Print and shaded views of the part. All mm, measured from the part's lowest x, y and z. Round coordinates to 2 decimals unless told otherwise and drop trailing zeros. Loops run counter-clockwise (first coordinate to the right, second up) from the corner with the lowest first, then second, coordinate; pieces in that order, holes last. Notation, with made-up numbers: (46.5, 58) - (66.5, 58) arc R27 ccw to (66.5, 92) - close; hole circle Ø10 at (85.25, 1). An arc over 180 degrees is marked (long way). Answer as a JSON object with one key per item and string values.
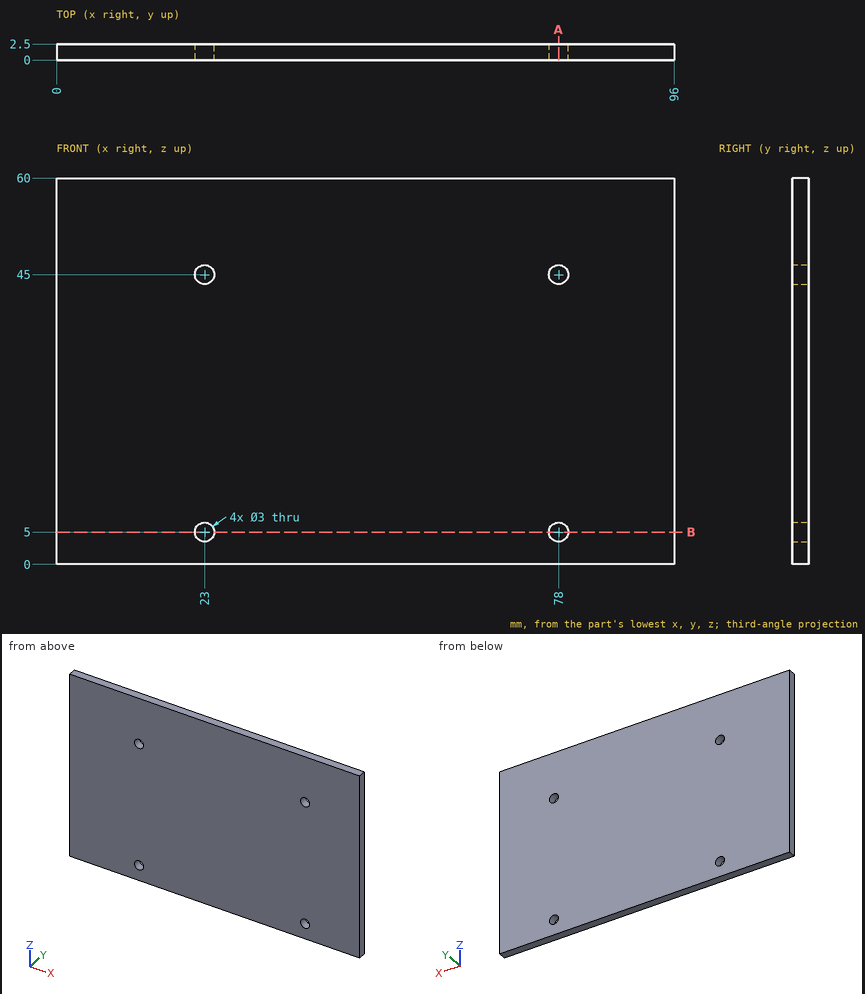
1) Probe probe 1 along Z at (x, y) = (78, 1.6); probe 2 along X at (y, z) = (0.75, 4). List the from-to ranges inside material, lowest first.
Values follow:
{"probe 1": "0 to 3.5, 6.5 to 43.5, 46.5 to 60", "probe 2": "0 to 21.88, 24.12 to 76.88, 79.12 to 96"}
2) Slice it at B-B on z = 5. List the corners of the cut face in (x, y).
Values follow:
{"outline": "(0, 0) - (21.5, 0) - (21.5, 2.5) - (0, 2.5) - close; (24.5, 0) - (76.5, 0) - (76.5, 2.5) - (24.5, 2.5) - close; (79.5, 0) - (96, 0) - (96, 2.5) - (79.5, 2.5) - close"}
3) Slice it at A-A on x = 78. List the corners of the cut face in (y, z), then the cut area to 3 significant figures.
Values follow:
{"outline": "(0, 0) - (2.5, 0) - (2.5, 3.5) - (0, 3.5) - close; (0, 6.5) - (2.5, 6.5) - (2.5, 43.5) - (0, 43.5) - close; (0, 46.5) - (2.5, 46.5) - (2.5, 60) - (0, 60) - close", "area": "135 mm²"}
4) Drop a flat-ended pin along its axis: P1, Ø2.5, axis at x = 78, z = 45, coming from the +Y side. Give the stop position or say it passes through.
Values follow:
{"P1": "through"}
